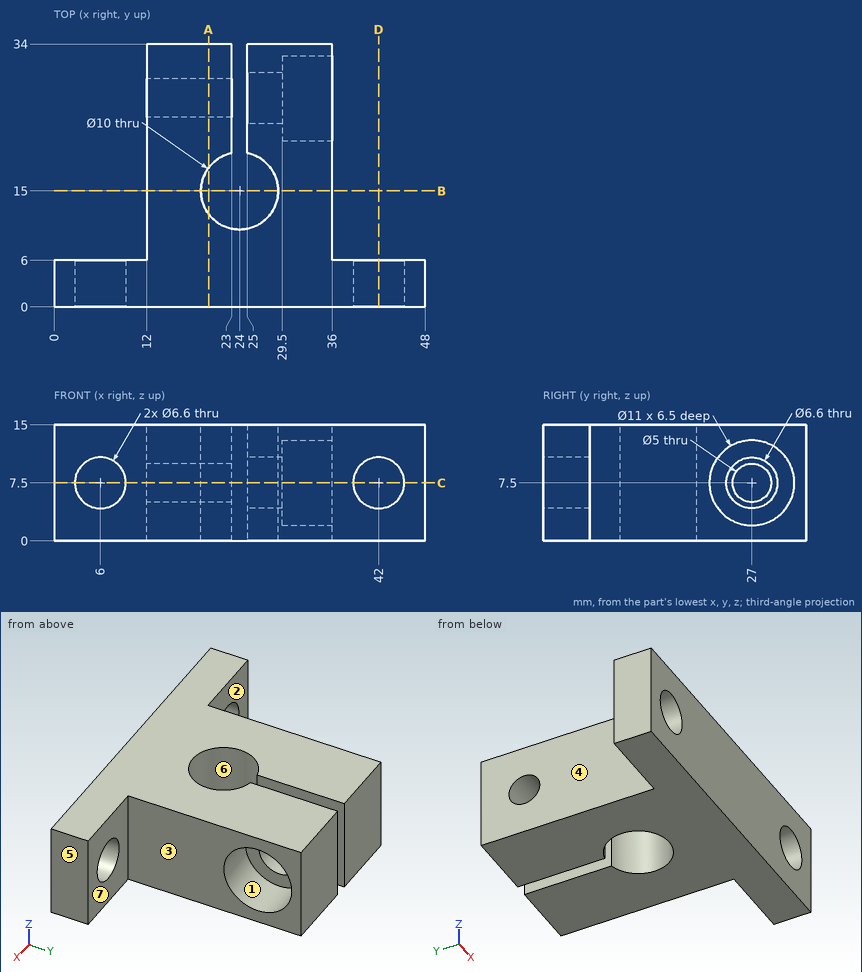
Check sheet for the drawn part. Datum: minimum x, y, z corner. Units: mm. A direction names the side the tool comes from. Round coordinates to 2 decimals unless told otherwise and drop trailing zeros. Loops run counter-clockwise (first coordinate to the right, second up) from the corner with the lowest first, then second, coordinate; pieces in that order, holes last. Notation, with made-up numbers: (80.25, 53) -> (101.25, 53) arc R21 ccw to (101.25, 66) -> close; hole circle Ø4 at (25.25, 2.25). An arc over 180 degrees is marked (long way). Put each result on its own line as item: value. Start each with the question number.
1. Section check C-C (z = 7.5). Give the number of separate pieces and of enclosed holes in the cut face, plus the area to 3 significant figures.
2. Section check A-A (x = 20). Enter the section's corners in (y, z).
3. Draft check along X on the marked faces 4, 5, 6 and 7. Enter one of: +X half, -X half, draft (parallel to the pull), parting line (faces both ways), or undercut.
4. Section check B-B (y = 15). Enter the section's corners in (x, z).
5. Scan lines: probe 1 along Z at (x, y) = (42, 3.1); probe 2 along Y at (x, z) = (32.25, 7.5); probe 3 along X at (y, z) = (21, 1.5). Record each from-to range of solid material in increasing order.
6. Section check D-D (x = 42). Enter the section's corners in (y, z).
7. Access from +Z, -Z, +X, -X, +Y, -Y to the whole of each face (thin tool, end or side, straight path). Record for the marked faces 1, 2 and 3.
8. Gauge pin test, flat ends, axial feed: pin 1 (6 mm diameter, centred on x = 42, z = 7.5, fed in from -Y); pin 2 (2 mm diameter, centred on x = 6, z = 2, fed in from -Y); pin 3 (1.5 mm diameter, centred on y = 17.5, z = 13, fed in from +X); pin 4 (4 mm diameter, centred on y = 25, z = 11, fed in from -X). Record the tip position at first contact, or that the pin passes through.
Findings:
1. separate pieces: 5
1. enclosed holes: 0
1. area: 618 mm^2
2. outline: (0, 0) -> (12, 0) -> (12, 15) -> (0, 15) -> close; (18, 0) -> (34, 0) -> (34, 15) -> (18, 15) -> close; hole circle Ø5 at (27, 7.5)
3. face 4: -X half
3. face 5: +X half
3. face 6: undercut
3. face 7: draft
4. outline: (12, 0) -> (19, 0) -> (19, 15) -> (12, 15) -> close; (29, 0) -> (36, 0) -> (36, 15) -> (29, 15) -> close
5. probe 1: z = 0 to 4.2, 10.8 to 15
5. probe 2: y = 0 to 21.5, 32.5 to 34
5. probe 3: x = 12 to 23, 25 to 36
6. outline: (0, 0) -> (6, 0) -> (6, 4.2) -> (0, 4.2) -> close; (0, 10.8) -> (6, 10.8) -> (6, 15) -> (0, 15) -> close
7. face 1: +X
7. face 2: +Z, -Z, -X, +Y
7. face 3: +Z, -Z, +X, +Y
8. pin 1: passes through
8. pin 2: stops at y = 0
8. pin 3: stops at x = 36
8. pin 4: stops at x = 12
